Part model, mm, in its own coordinate system. A direction names the side the tool comes from. Give positions to 0.01 mm unless a question says otherwise; leave off trailing zeros. Write each loop counter-clockwise with the first axis right and the second up, starting at its lowest first coordinate (ties: lowest second). Pieces come first, ordered by that corner, then holes. Notation, with made-up numbers: M 66.25,19.25 L 121.25,19.25 A13 cw 121.25,34.25 Z; hole C 45,-3 d5. An arc over 180 degrees is marked long. Answer as CSV lines item,"result". Start each with the question number.
Item 1: 3-axis set-ups, long thin cutter, end or side, ignore diameter. For faces 1 (the flat face through (-31, 12, 47)), 2 (the flat face through (-21, 21, 0)): which of +Z, -Z, +X, -X, +Y, -Y reach the whole face in a straight line?
Item 2: Band-saw the part on A-A, the plane x = -13. List the corners of the cut face in (y, z).
Item 3: Band-saw the part on B-B, the plane y = 14.5. List the corners of the cut face in (x, z), then the cut area to 3 significant figures.
Item 4: Wall check: L1, parallel to Z at x = -14, y = 24; L2, parallel to Z at x = -29, y = 4; L3, parallel to X at y = 20, z = 237.5. Give the ranges that are in metal, low to high. Write a range as from..to.
Item 5: Band-saw the part on C-C, the plane z = 52.5. List the corners of the cut face in (x, y).
Item 6: Pin check, flat tips, straight feed: pin 1 (10 mm diameter, centred on y = 9.5, z = 199, fed in from -X); pin 2 (1 mm diameter, centred on x = -22, y = 34.5, fed in from +Z); pin 3 (6.5 mm diameter, centred on x = -26.5, y = 19, fed in from +Z). Stop position of each tip, or through.
from build123d import *

# Parameters (mm, degrees)
SKETCH_1_W      = 42
SKETCH_1_H      = 42
EXTRUDE_1_DEPTH = 47
CHAMFER_1_SIZE  = 3
SKETCH_2_R      = 11
EXTRUDE_2_DEPTH = 2
SKETCH_3_R      = 2.5
EXTRUDE_3_DEPTH = 300


with BuildPart() as part:
    # 草图1 → 凸台-拉伸1 (new body)
    with BuildSketch(Plane.XY):
        with Locations((-21, 21)):
            Rectangle(SKETCH_1_W, SKETCH_1_H)
    extrude(amount=EXTRUDE_1_DEPTH)

    # 倒角1
    chamfer_1_edges = [part.edges().sort_by_distance(p)[0] for p in [
        (0, 0, 23.5),
        (-42, 0, 23.5),
        (-42, 42, 23.5),
        (0, 42, 23.5),
    ]]
    chamfer(chamfer_1_edges, length=CHAMFER_1_SIZE)

    # 草图2 → 凸台-拉伸2 (add)
    with BuildSketch(Plane.XY.offset(47)):
        with Locations((-21, 21)):
            Circle(SKETCH_2_R)
    extrude(amount=EXTRUDE_2_DEPTH)

    # 草图3 → 凸台-拉伸3 (add)
    with BuildSketch(Plane.XY.offset(49)):
        with Locations((-21, 21)):
            Circle(SKETCH_3_R)
    extrude(amount=EXTRUDE_3_DEPTH)


solid = part.part
Output:
1,face 1,"+Z"
1,face 2,"-Z, +X, -X, +Y, -Y"
2,outline,"M 0,0 L 42,0 L 42,47 L 28.55,47 L 28.55,49 L 13.45,49 L 13.45,47 L 0,47 Z"
3,outline,"M -42,0 L 0,0 L 0,47 L -12.13,47 L -12.13,49 L -29.87,49 L -29.87,47 L -42,47 Z"
3,area,"2,010 mm²"
4,L1,"0..49"
4,L2,"0..47"
4,L3,"-23.29..-18.71"
5,outline,"C -21,21 d5"
6,pin 1,"through"
6,pin 2,"z = 47"
6,pin 3,"z = 49"
